Build history of the part. All positions in model axes, mm. Face numbers are marked on the shaded views. A direction names the side the tool comes from. Round coordinates to 2 decimals unless told otherwise and drop trailing zeros. Order: outer loops, then holes, each group sorted by start corner. A loop starts at its lowest first (then second) coordinate and runs counter-clockwise, first axis right, second up. Notation, with made-up numbers: (-12.75, -37) -> (23.25, -37) arc R23 ccw to (23.25, -21) -> close; hole circle Ø5 at (-26, 36). An arc over 180 degrees is marked (long way). Use a Markdown table: item, result. Add a question column.
Item 1: Pin check, flat tips, straight feed: pin 1 (1 mm diameter, centred on y = -1, z = 62.5, fed in from +X); pin 2 (3.5 mm diameter, centred on x = 39, z = 10, fed in from +Y); pin 3 (1.5 mm diameter, centred on x = -6, z = 89, fed in from +Y); pin 4 (2 mm diameter, centred on x = 36.5, y = -1.5, fed in from -Z). Stop position of each tip, or through.
Item 2: Slice it at D-D, the plane z = 110. Give the cut face in (x, y).
Item 3: 3-axis set-ups, long thin cutter, end or side, ignore diameter. For the marked faces 1 and 2: which of +Z, -Z, +X, -X, +Y, -Y reach the whole face in a straight line?
Item 4: Slice it at B-B, the plane z = 10. Give the cut face in (x, y).
Item 5: Slice it at C-C, the plane x = 39. Give the cut face in (y, z).
Item 6: Probe L1, parallel to Z at x = 39, y = -1.15; L2, parallel to Y at x = 24, z = 18; L3, parallel to X at y = -0.55, z = 110. List the from-to ranges inside material, lowest first.
Item 7: Slice it at A-A, the plane x = 31. Give the cut face in (y, z).
from build123d import *

# Parameters (mm, degrees)
F1_DEPTH = 120
F6_R     = 1.5
F6_W     = 25
F6_H     = 74
F2_DEPTH = 2.001
F6_W_2   = 2
F6_H_2   = 120
F3_DEPTH = 3
F4_W     = 11
F4_H     = 21
F5_DEPTH = 25


with BuildPart() as f1:
    # F0 (on Top) → F1 (new body)
    with BuildSketch(Plane.XY):
        Polygon((45, 0), (0, 0), (-32.1393804843, 38.3022221559), (-33.6714693706, 37.0166469366), (0, -2), (45, -2), align=None)
    extrude(amount=F1_DEPTH)

    # F6 (on face) → F2 (cut, through all)
    with BuildSketch(Plane(origin=(0, 0, 0), x_dir=(-1, 0, 0), z_dir=(0, 1, 0))):
        with Locations((-39, 110)):
            Circle(F6_R)
        with Locations((-39, 10)):
            Circle(F6_R)
        with Locations((-32.5, 60)):
            Rectangle(F6_W, F6_H)
    extrude(amount=-F2_DEPTH, mode=Mode.SUBTRACT)

    # F6 (on face) → F3 (join)
    with BuildSketch(Plane(origin=(0, 0, 0), x_dir=(-1, 0, 0), z_dir=(0, 1, 0))):
        with Locations((-10.4, 60)):
            Rectangle(F6_W_2, F6_H_2)
    extrude(amount=F3_DEPTH)

    # F4 (on face) → F5 (cut)
    with BuildSketch(Plane(origin=(0, 0, 0), x_dir=(-0.6427876097, 0.7660444431, 0), z_dir=(0.7660444431, 0.6427876097, 0))):
        with Locations((18.5, 10.5)):
            Rectangle(F4_W, F4_H)
    extrude(amount=-F5_DEPTH, mode=Mode.SUBTRACT)


solid = f1.part
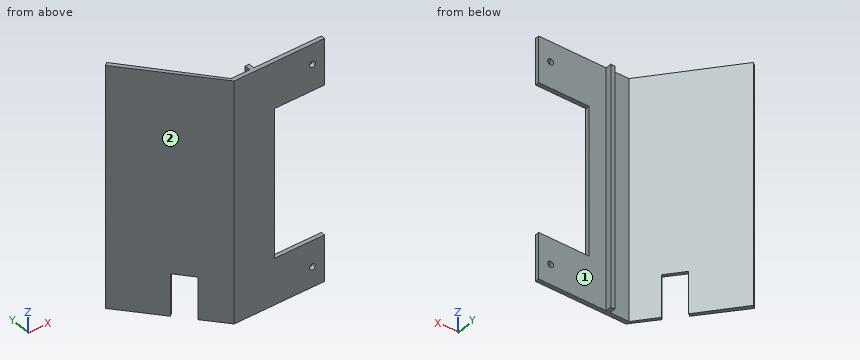
Check sheet entries:
| question | item | result |
|---|---|---|
| 1 | pin 1 | x = 20 |
| 1 | pin 2 | y = 0 |
| 1 | pin 3 | y = 8.04 |
| 1 | pin 4 | z = 0 |
| 2 | outline | (-33.67, 37.02) -> (0, -2) -> (37.5, -2) -> (37.5, 0) -> (11.4, 0) -> (11.4, 3) -> (9.4, 3) -> (9.4, 0) -> (0, 0) -> (-32.14, 38.3) -> close; (40.5, -2) -> (45, -2) -> (45, 0) -> (40.5, 0) -> close |
| 3 | face 1 | +Z, -Z, +X, +Y |
| 3 | face 2 | +Z, -Z, -X, -Y |
| 4 | outline | (-33.67, 37.02) -> (-16.68, 17.33) -> (-15.43, 18.39) -> (-32.14, 38.3) -> close; (-9.5, 9) -> (0, -2) -> (37.5, -2) -> (37.5, 0) -> (11.4, 0) -> (11.4, 3) -> (9.4, 3) -> (9.4, 0) -> (0, 0) -> (-8.36, 9.96) -> close; (40.5, -2) -> (45, -2) -> (45, 0) -> (40.5, 0) -> close |
| 5 | outline | (-2, 0) -> (0, 0) -> (0, 8.5) -> (-2, 8.5) -> close; (-2, 11.5) -> (0, 11.5) -> (0, 23) -> (-2, 23) -> close; (-2, 97) -> (0, 97) -> (0, 108.5) -> (-2, 108.5) -> close; (-2, 111.5) -> (0, 111.5) -> (0, 120) -> (-2, 120) -> close |
| 6 | L1 | 0 to 8.5, 11.5 to 23, 97 to 108.5, 111.5 to 120 |
| 6 | L2 | -2 to 0 |
| 6 | L3 | -1.25 to 37.5, 40.5 to 45 |
| 7 | outline | (-2, 0) -> (0, 0) -> (0, 23) -> (-2, 23) -> close; (-2, 97) -> (0, 97) -> (0, 120) -> (-2, 120) -> close |
